from build123d import *

# Parameters (mm, degrees)
CYLINDER111_R     = 1.6
CYLINDER111_DEPTH = 15


with BuildPart() as cylinder111:
    # Cylinder111 → Cylinder111 (new body)
    with BuildSketch(Plane.XY):
        Circle(CYLINDER111_R)
    extrude(amount=CYLINDER111_DEPTH)


with BuildPart() as fusion045:
    # Cone013 → Cone013 (revolve)
    with BuildSketch(Plane(origin=(0, 0, 15), x_dir=(1, 0, 0), z_dir=(0, -1, 0))):
        Polygon((0, 0), (1.6, 0), (3, 3.5), (0, 3.5), align=None)
    revolve(axis=Axis((0, 0, 15), (0, 0, 1)))

    # Fusion045: union Cylinder111
    add(cylinder111.part)


with BuildPart() as fusion045_1:
    # Fusion045 placement: moved
    add(fusion045.part.moved(Location((118.9, 37.2, 48.8))))


solid = fusion045_1.part
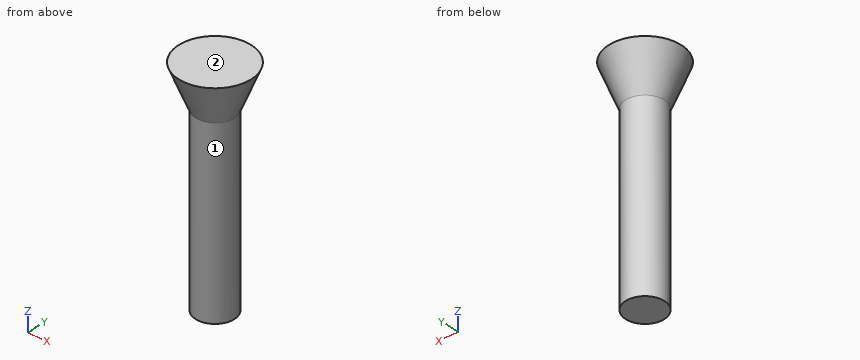
Design review of the part built by this model. Coordinates are the model's own, in mm. Face numbers are marked on the shaded views. A direction names the side the tool comes from. Round coordinates to 2 decimals unless told otherwise and drop trailing zeros. Write each loop counter-clockwise with the first axis right and the second up, starting at its lowest first coordinate (ties: lowest second). Pieces come first, ordered by that corner, then holes. Notation, with made-up numbers: (50, 57) - (80, 57) arc R12 ccw to (80, 68) - close; hole circle Ø6 at (43, 7.25). An arc over 180 degrees is marked (long way). Return JSON: item names as keys, results as strings. Group by question number.
Item 1: Machinability: for the marked faces 1 and 2, which of the approach directions +Z, -Z, +X, -X, +Y, -Y give a long, thin tool a straight path to every point of the face, cutting with its end or side? Answer none if there is none.
Item 2: Insertion check: P1, Ø2, axis at y = 39.5, z = 57, coming from the -X side; P2, Ø3, axis at y = 38.5, z = 59.5, coming from the -X side; P3, Ø1.5, axis at y = 38, z = 54.5, coming from the +X side. Each pin has a flat end and moves straight along its axis. Give the tip position at first contact, or say it passes through.
Item 3: We need section B-B on y = 37.2. Write out the cut boundary in (x, z).
Item 4: We need section A-A on x = 118.9. Write out the cut boundary in (y, z).
Item 5: For probe 1 along X at (y, z) = (37.15, 50.5); probe 2 along X at (y, z) = (38.55, 61); probe 3 along Z at (x, y) = (119.45, 39), list the stretches that pass through material, from the lowest coordinate up. Write a range as [from, to].
Item 6: We need section C-C on z = 61.25. Write out the cut boundary in (x, y), and give its area (3 significant figures).
Model answer:
{
 "1": {"face 1": "-Z", "face 2": "+Z, +X, -X, +Y, -Y"},
 "2": {"P1": "stops at x = 117.97", "P2": "stops at x = 117.3", "P3": "stops at x = 120.5"},
 "3": {"outline": "(115.9, 67.3) - (117.3, 63.8) - (117.3, 48.8) - (120.5, 48.8) - (120.5, 63.8) - (121.9, 67.3) - close"},
 "4": {"outline": "(34.2, 67.3) - (35.6, 63.8) - (35.6, 48.8) - (38.8, 48.8) - (38.8, 63.8) - (40.2, 67.3) - close"},
 "5": {"probe 1": "x = [117.3, 120.5]", "probe 2": "x = [118.04, 119.76]", "probe 3": "z = [64.51, 67.3]"},
 "6": {"outline": "circle Ø3.2 at (118.9, 37.2)", "area": "8.04 mm²"}
}
